```python
from build123d import *

# Parameters (mm, degrees)
F0_W     = 838.2
F0_H     = 409.575
F1_DEPTH = 12.7
F7_DEPTH = 6.35


with BuildPart() as f1:
    # F0 (on Top) → F1 (new body)
    with BuildSketch(Plane.XY):
        Rectangle(F0_W, F0_H)
    extrude(amount=F1_DEPTH)

    # F4: sweep along a path in F2
    with BuildLine(Plane(origin=(0, 0, 0), x_dir=(1, 0, 0), z_dir=(0, 0, -1))) as f4_path:
        Line((339.725, 204.7875), (339.725, -89.8525))
        ThreePointArc((339.725, -89.8525), (321.8702293811, -132.9577293811), (278.765, -150.8125))
        Line((278.765, -150.8125), (-278.765, -150.8125))
    # F3 (on face) → F4 (sweep, cut)
    with BuildSketch(Plane.XZ.offset(204.7875)):
        with BuildLine():
            Line((419.1, 0), (419.1, 6.35))
            Line((419.1, 6.35), (346.075, 6.35))
            ThreePointArc((346.075, 6.35), (342.4088257906, 5.1847532889), (340.088162586, 2.1166666667))
            ThreePointArc((340.088162586, 2.1166666667), (338.9278309836, 0.5826233556), (337.0947438789, 0))
            Line((337.0947438789, 0), (419.1, 0))
        make_face()
        Polygon((419.1, -8.3515942097), (419.1, 0), (337.0947438789, 0), (334.0992927551, 0), (334.0992927551, -8.3515942097), align=None)
    sweep(path=f4_path.line, mode=Mode.SUBTRACT)

    # F5: sweep along a path in F2
    with BuildLine(Plane(origin=(0, 0, 0), x_dir=(1, 0, 0), z_dir=(0, 0, -1))) as f5_path:
        Line((-339.725, 204.7875), (-339.725, -89.8525))
        ThreePointArc((-339.725, -89.8525), (-321.8702293811, -132.9577293811), (-278.765, -150.8125))
    # F3 (on face) → F5 (sweep, cut)
    with BuildSketch(Plane.XZ.offset(204.7875)):
        Polygon((-334.0992927551, -8.3515942097), (-334.0992927551, 0), (-337.0947438789, 0), (-419.1, 0), (-419.1, -8.3515942097), align=None)
        with BuildLine():
            Line((-346.075, 6.35), (-419.1, 6.35))
            Line((-419.1, 6.35), (-419.1, 0))
            Line((-419.1, 0), (-337.0947438789, 0))
            ThreePointArc((-337.0947438789, 0), (-338.9278309836, 0.5826233556), (-340.088162586, 2.1166666667))
            ThreePointArc((-340.088162586, 2.1166666667), (-342.4088257906, 5.1847532889), (-346.075, 6.35))
        make_face()
    sweep(path=f5_path.line, mode=Mode.SUBTRACT)

    # F6 (on face) → F7 (cut)
    with BuildSketch(Plane(origin=(0, 0, 0), x_dir=(1, 0, 0), z_dir=(0, 0, -1))):
        Polygon((-393.2344317436, -48.8721951842), (-452.7488350868, -48.8721951842), (-471.2188243866, -238.360658288), (-328.9314508438, -230.1517724991), align=None)
        Polygon((437.9153549671, 9.2740878463), (311.3617002964, -234.2562228441), (450.2286911011, -257.5147151947), align=None)
    extrude(amount=-F7_DEPTH, mode=Mode.SUBTRACT)


solid = f1.part
```
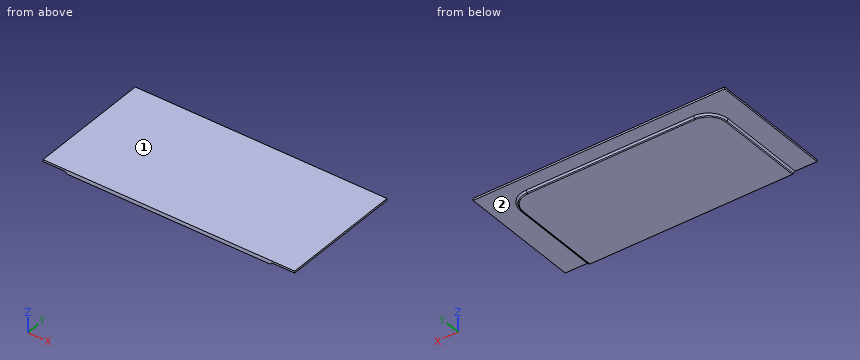
Verification items for the finished model (mm, model axes). Face numbers are marked on the shaded views. A direction names the side the tool comes from. Coordinates: 2 decimals unless noted, no trailing zeros. Loops run counter-clockwise (first coordinate to the right, second up) from the corner with the lowest first, then second, coordinate; pieces in that order, holes last. Notation, with made-up numbers: (79, -11.5) -> (136, -11.5) arc R22 cw to (136, 17.5) -> close; hole circle Ø8 at (9.5, 76). An arc over 180 degrees is marked (long way). Answer in a Markdown table with one row per item.
1) Depth check by flat-ended pin: P1, Ø1, axis at y = -93, z = 3, coming from the -X side; P2, Ø1.5, axis at x = -84, z = 6, coming from the +Y side. Enter the tip coordinate at first touch or a pass-through.
The answers:
| item | result |
|---|---|
| P1 | stops at x = -340.78 |
| P2 | stops at y = 204.79 |
2) Section check A-A (y = -57). Record the cut outline in (x, z) (3 decimals), and give its area (3 significant figures).
The answers:
| item | result |
|---|---|
| outline | (-419.1, 6.35) -> (-346.075, 6.35) arc R6.35 cw to (-340.088, 2.117) arc R3.175 ccw to (-337.095, 0) -> (337.095, 0) arc R3.175 ccw to (340.088, 2.117) arc R6.35 cw to (346.075, 6.35) -> (419.1, 6.35) -> (419.1, 12.7) -> (-419.1, 12.7) -> close |
| area | 9,650 mm2 |
3) Access from +Z, -Z, +X, -X, +Y, -Y to the whole of each face (thin tool, end or side, straight path). Record for the marked faces 1 and 2.
The answers:
| item | result |
|---|---|
| face 1 | +Z, +X, -X, +Y, -Y |
| face 2 | -Z, +Y |
4) Scan lines: line 1 along Y through (x, z) = (-88, 2); line 2 along Z through (x, y) = (368, 83.5); line 3 along Y through (x, z) = (-159.5, 1.75). Record each from-to range of solid material in increasing order. Write a range as from..to.
The answers:
| item | result |
|---|---|
| line 1 | y = -204.79..151.13 |
| line 2 | z = 6.35..12.7 |
| line 3 | y = -204.79..151.02 |
